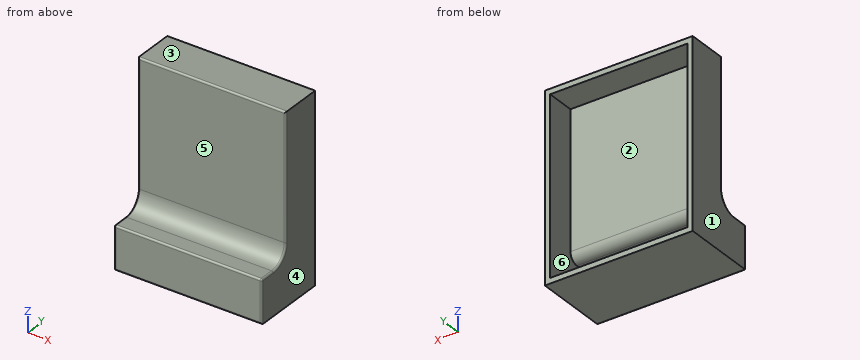
```python
from build123d import *

# Parameters (mm, degrees)
SKETCH_W        = 82.5
SKETCH_H        = 104
PAD_DEPTH       = 23
SKETCH001_W     = 76.6
SKETCH001_H     = 98
POCKET_DEPTH    = 16
SKETCH002_W     = 82.5
SKETCH002_H     = 24
PAD001_DEPTH    = 19
FILLET_R        = 10
FILLET001_R     = 1
FILLET002_R     = 1
SKETCH003_W     = 76.6
SKETCH003_H     = 17
POCKET001_DEPTH = 21
FILLET003_R     = 5


with BuildPart() as part:
    # Sketch → Pad (new body)
    with BuildSketch(Plane.XZ):
        Rectangle(SKETCH_W, SKETCH_H)
    extrude(amount=PAD_DEPTH)

    # Sketch001 → Pocket (cut)
    with BuildSketch(Plane.XZ):
        Rectangle(SKETCH001_W, SKETCH001_H)
    extrude(amount=POCKET_DEPTH, mode=Mode.SUBTRACT)

    # Sketch002 → Pad001 (join)
    with BuildSketch(Plane(origin=(0, -23, 1), x_dir=(1, 0, 0), z_dir=(0, -1, 0))):
        with Locations((0, -41)):
            Rectangle(SKETCH002_W, SKETCH002_H)
    extrude(amount=PAD001_DEPTH)

    # Fillet
    fillet_edges = [part.edges().sort_by_distance(p)[0] for p in [
        (0, -23, -28),
    ]]
    fillet(fillet_edges, radius=FILLET_R)

    # Fillet001
    fillet001_edges = [part.edges().sort_by_distance(p)[0] for p in [
        (41.25, -23, 17),
        (0, -23, 52),
        (-41.25, -23, 17),
    ]]
    fillet(fillet001_edges, radius=FILLET001_R)

    # Fillet002
    fillet002_edges = [part.edges().sort_by_distance(p)[0] for p in [
        (0, -42, -28),
        (-40.957107, -42, -28.292893),
        (40.957107, -42, -28.292893),
        (-41.25, -42, -40.5),
        (41.25, -42, -40.5),
        (0, -42, -52),
    ]]
    fillet(fillet002_edges, radius=FILLET002_R)

    # Sketch003 → Pocket001 (cut)
    with BuildSketch(Plane.XZ.offset(16)):
        with Locations((0, -40.5)):
            Rectangle(SKETCH003_W, SKETCH003_H)
    extrude(amount=POCKET001_DEPTH, mode=Mode.SUBTRACT)

    # Fillet003
    fillet003_edges = [part.edges().sort_by_distance(p)[0] for p in [
        (0, -16, -32),
    ]]
    fillet(fillet003_edges, radius=FILLET003_R)


solid = part.part
```
Input: part model. Units: mm. Frame: model coordinates. Face numbers are marked on the shaded views. A direction names the side the tool comes from. Round coordinates to 2 decimals unless told otherwise and drop trailing zeros. Loops run counter-clockwise (first coordinate to the right, second up) from the corner with the lowest first, then second, coordinate; pieces in that order, holes last. Notation, with made-up numbers: (-9, 85) -> (7, 85) arc R15 ccw to (7, 109) -> close; hole circle Ø6 at (64.5, 26.5). An arc over 180 degrees is marked (long way). Use one line per item in the form item = value. Start each with the question number.
Item 1: Mould query, pull axis X, two halves, no side actions, for the marked faces 1, 2 and 3. Classes: pulls with the +X half, pulls with the -X half, needs draft (parallel to the pull), parting line crosses it, or undercut.
Item 2: Contact query for flat-ended pins moving along their axis: pin 1 Ø3 at (x, y) = (-4, -27) entering from +Z; pin 2 Ø6.5 at (x, y) = (-4.5, -36) entering from +Z; pin 3 Ø23 at (x, z) = (16, -3.5) entering from +Y. Output: stop coordinate, or through.
Item 3: Set-up query: the marked faces 4, 5 and 6. Return all of +Z, -Z, +X, -X, +Y, -Y with unobstructed straight access to the full face (end or side cutting, diameter ignored); none if empty.
Item 4: Section query C-C on x = -34.5. Return the cut outline in (y, z), then the cut area to 3 significant figures.
Item 5: Section query D-D on z = -35.5. Return the cut outline in (x, y), then the cut area to 3 significant figures.
Item 6: Section query A-A on y = -12.5. Return the cut outline in (x, z), then the cut area to 3 significant figures.
Item 7: Material intervals for L1, parallel to X at y = -4.5, z = -23.5; L2, parallel to Z at x = -10, y = -15.5; L3, parallel to Z at x = -1, y = -22, sorted ascending. Write a range as from..to.
Item 8: Section query B-B on z = 13.5. Return the cut outline in (x, y), then the cut area to 3 significant figures.
Ans:
q1.face_1 = pulls with the -X half
q1.face_2 = undercut
q1.face_3 = needs draft
q2.pin_1 = -24.61
q2.pin_2 = -28
q2.pin_3 = -16
q3.face_4 = +Z, -Z, +X, +Y, -Y
q3.face_5 = +Z, +X, -X, -Y
q3.face_6 = +Y
q4.outline = (-42, -51) arc R1 ccw to (-41, -52) -> (0, -52) -> (0, -49) -> (-37, -49) -> (-37, -32) -> (-21, -32) arc R5 ccw to (-16, -27) -> (-16, 49) -> (0, 49) -> (0, 52) -> (-22, 52) arc R1 ccw to (-23, 51) -> (-23, -18) arc R10 cw to (-33, -28) -> (-41, -28) arc R1 ccw to (-42, -29) -> close
q4.area = 938 mm^2
q5.outline = (-41.25, -41) arc R1 ccw to (-40.25, -42) -> (40.25, -42) arc R1 ccw to (41.25, -41) -> (41.25, 0) -> (38.3, 0) -> (38.3, -37) -> (-38.3, -37) -> (-38.3, 0) -> (-41.25, 0) -> close
q5.area = 630 mm^2
q6.outline = (-41.25, -52) -> (41.25, -52) -> (41.25, 52) -> (-41.25, 52) -> close; hole (-38.3, -49) -> (38.3, -49) -> (38.3, 49) -> (-38.3, 49) -> close
q6.area = 1,070 mm^2
q7.L1 = -41.25..-38.3, 38.3..41.25
q7.L2 = -52..-49, 49..52
q7.L3 = -52..-49, -32..52
q8.outline = (-41.25, -22) arc R1 ccw to (-40.25, -23) -> (40.25, -23) arc R1 ccw to (41.25, -22) -> (41.25, 0) -> (38.3, 0) -> (38.3, -16) -> (-38.3, -16) -> (-38.3, 0) -> (-41.25, 0) -> close
q8.area = 671 mm^2
